Could you check a few things on this model? Use its own coordinates, in mm. A direction names the side the tool comes from. Give positions to 0.01 mm unless a question says otherwise; leave off trailing zeros. Write each loop counter-clockwise with the first axis right and the second up, starting at its lowest first coordinate (ties: lowest second). Pieces come first, ordered by that corner, then holes. Notation, with made-up numbers: (76, 16) - (98, 16) arc R6 ccw to (98, 23) - close; hole circle Ø6 at (89, 67). An arc over 180 degrees is marked (long way). Answer as CSV lines item,"result". Start each with the question number.
Q1. We'd pull the mould along X, two halves only. Please class faces 1 (the face through (-25.46, 12.54, -32.66)), 2 (the face through (-26.55, 17.465, -29.405)), 3 (the face through (-18, 17, -26.94)), 4 (the face through (-25.46, 22.54, -32.66)): pulls with the +X half, pulls with the -X half, needs draft (parallel to the pull), parting line crosses it, or undercut.
Q2. Will these pins go through, and if not, where does the flat tip stop? pin 1 Ø9.5 at (x, z) = (-48.5, -28) entering from +Y; pin 2 Ø8 at (x, z) = (-19.5, -31) entering from +Y; pin 3 Ø3 at (x, z) = (-45, -29) entering from -Y; pin 4 Ø4 at (x, z) = (-22.24, -31.94) entering from -Y.
Q3. If I drill on line 1 along Y through (x, z) = (-16, -34.5); line 2 along Z through (x, y) = (-20, 10.5); line 3 along X through (y, z) = (21.75, -26), over which ranges is the centre line in solid material (lowest first)?
Q4. On a 3-axis mill with a long thin cutter (end or side, diameter ignored), from which of +Z, -Z, +X, -X, +Y, -Y can I reach the whole of each face in a straight line? I mean faces 5 (the face through (-18, 17, -36.94)), 6 (the face through (-31, 12, -16.94)), 7 (the face through (-38.032, 22.535, -26.833)). Say none if no direction works.
Q5. Imagine slicing it at D-D on x = -54. List the corners of the cut face in (y, z) for me, and give its area (3 significant figures).
Q6. Imagine slicing it at C-C on y = 18.75. List the corners of the cut face in (x, z) for me, and give its area (3 significant figures).
Q7. Imagine slicing it at B-B on x = -16. List the corners of the cut face in (y, z) for me, and give its area (3 significant figures).
Q8. Imagine slicing it at A-A on z = -34. State how many separate pieces and enclosed holes the cut face has, and give its area (3 significant figures).
```python
from build123d import *

# Parameters (mm, degrees)
ESQUISSE1_W                = 50
ESQUISSE1_H                = 30
BOSS_EXTRU_1_DEPTH         = 25
ESQUISSE2_R                = 9.5
ENL_V_MAT_EXTRU_1_DEPTH    = 5
ESQUISSE5_R                = 3.3
ENL_V_MAT_EXTRU_2_DEPTH    = 30
ENL_V_MAT_EXTRU_3_DEPTH    = 30
CONG_1_R                   = 10
ENL_V_START                = -5
ESQUISSE8_R                = 3.3
ENL_V_MAT_EXTRU_4_DEPTH    = 5
R_P_TITION_LIN_AIRE1_COUNT = 2
R_P_TITION_LIN_AIRE1_PITCH = 10


with BuildPart() as part:
    # Esquisse1 → Boss.-Extru.1 (new body)
    with BuildSketch(Plane(origin=(0, 0, 0), x_dir=(1, 0, 0), z_dir=(0, 1, 0))):
        with Locations((-35.541978222, 31.940035978)):
            Rectangle(ESQUISSE1_W, ESQUISSE1_H)
    extrude(amount=BOSS_EXTRU_1_DEPTH)

    # Esquisse2 → Enlèv. mat.-Extru.1 (cut)
    with BuildSketch(Plane(origin=(0, 25, 0), x_dir=(1, 0, 0), z_dir=(0, 1, 0))):
        with Locations(Location((-46.041978222, 31.940035978, 0), (0, 0, 270))):  # turned: the seam where the file's is
            Circle(ESQUISSE2_R)
    extrude(amount=-ENL_V_MAT_EXTRU_1_DEPTH, mode=Mode.SUBTRACT)

    # Esquisse5 → Enlèv. mat.-Extru.2 (cut)
    with BuildSketch(Plane(origin=(0, 25, 0), x_dir=(1, 0, 0), z_dir=(0, 1, 0))):
        with Locations(Location((-22.240136575, 31.940035978, 0), (0, 0, 270))):  # turned: the seam where the file's is
            Circle(ESQUISSE5_R)
    extrude(amount=-ENL_V_MAT_EXTRU_2_DEPTH, mode=Mode.SUBTRACT)

    # Esquisse7 → Enlèv. mat.-Extru.3 (cut)
    with BuildSketch(Plane(origin=(0, 0, -46.940035978), x_dir=(-1, 0, 0), z_dir=(0, 0, -1))):
        Polygon((30.901738287, 0), (60.541978222, 12.5), (60.541978222, 0), align=None)
    extrude(amount=-ENL_V_MAT_EXTRU_3_DEPTH, mode=Mode.SUBTRACT)

    # Congé1
    cong_1_edges = [part.edges().sort_by_distance(p)[0] for p in [
        (-60.541978222, 18.75, -46.940035978),
        (-60.541978222, 18.75, -16.940035978),
    ]]
    fillet(cong_1_edges, radius=CONG_1_R)

    # Esquisse8 → Enlèv. mat.-Extru.4 (cut)
    with BuildSketch(Plane.XZ.offset(ENL_V_START)):
        Polygon((-25.12688792, -36.940035978), (-19.353385229, -36.940035978), (-16.466633883, -31.940035978), (-19.353385229, -26.940035978), (-25.12688792, -26.940035978), (-28.013639266, -31.940035978), align=None)
        with Locations(Location((-22.240136575, -31.940035978, 0), (0, 0, 90))):  # turned: the seam where the file's is
            Circle(ESQUISSE8_R, mode=Mode.SUBTRACT)
        Polygon((-16.466633883, -31.940035978), (-19.353385229, -36.940035978), (-10.541978222, -36.940035978), (-10.541978222, -26.940035978), (-19.353385229, -26.940035978), align=None)
    enl_v_mat_extru_4 = extrude(amount=-ENL_V_MAT_EXTRU_4_DEPTH, mode=Mode.SUBTRACT)

    # Répétition linéaire1: Enlèv. mat.-Extru.4 ×2
    with Locations(*[(0, i * R_P_TITION_LIN_AIRE1_PITCH, 0) for i in range(1, R_P_TITION_LIN_AIRE1_COUNT)]):
        add(enl_v_mat_extru_4, mode=Mode.SUBTRACT)


solid = part.part
```
Conclusion:
1,face 1,"undercut"
1,face 2,"pulls with the +X half"
1,face 3,"needs draft"
1,face 4,"undercut"
2,pin 1,"y = 20"
2,pin 2,"y = 25"
2,pin 3,"y = 5.31"
2,pin 4,"through"
3,line 1,"0 to 5, 10 to 15, 20 to 25"
3,line 2,"-46.94 to -34.36, -29.52 to -16.94"
3,line 3,"-60.5 to -53.46, -38.63 to -10.54"
4,face 5,"+X"
4,face 6,"+Z, +X, -X, +Y, -Y"
4,face 7,"+Y"
5,outline,"(9.74, -46.32) - (25, -46.32) - (25, -37.13) - (20, -37.13) - (20, -26.75) - (25, -26.75) - (25, -17.56) - (9.74, -17.56) - close"
5,area,"387 mm^2"
6,outline,"(-60.54, -36.94) arc R10 ccw to (-50.54, -46.94) - (-10.54, -46.94) - (-10.54, -36.94) - (-25.13, -36.94) - (-28.01, -31.94) - (-25.13, -26.94) - (-10.54, -26.94) - (-10.54, -16.94) - (-50.54, -16.94) arc R10 ccw to (-60.54, -26.94) - close"
6,area,"1,300 mm^2"
7,outline,"(0, -46.94) - (25, -46.94) - (25, -16.94) - (0, -16.94) - close; hole (5, -36.94) - (10, -36.94) - (10, -26.94) - (5, -26.94) - close; hole (15, -36.94) - (20, -36.94) - (20, -26.94) - (15, -26.94) - close"
7,area,"650 mm^2"
8,separate pieces,"4"
8,enclosed holes,"0"
8,area,"732 mm^2"
